Input: part model. Units: mm. Frame: model coordinates. A direction names the side the tool comes from. Round coordinates to 2 decimals unless told otherwise and drop trailing zeros. Loops run counter-clockwise (first coordinate to the right, second up) from the corner with the lowest first, then second, coordinate; pieces in that order, holes last.
1) First-contact query: pin 1 (0.9 mm diameter, centred on x = 0, y = 1, fed in from +Z); pin 2 (1 mm diameter, centred on x = 0.5, y = -1, fed in from +Z); pin 3 (0.9 mm diameter, centred on x = 0, y = -0.5, fed in from -Z); pin 4 (3 mm diameter, centred on y = -1, z = -1.5, fed in from +X). Flat tips, straight axial feed; report the tip coordinate or a pass-through.
2) Ray query, line 1 along Y through (x, z) = (0, -0.6); line 2 along Y through (x, z) = (-0.4, -1). Return the intervals inside material, ascending.
3) Section D-D, the plane z = -1. Return loops of the section in (x, y), and give its area (3 significant figures).
4) Access query for faces 5 (the face through (1, -0.7, 1.2)), 6 (the face through (-1, -0.7, 1.2)), 7 (the face through (-2.12, 1.17, 2.07)). Directions: +Z, -Z, +X, -X, +Y, -Y. A direction counts if a zero-diameter tool reaches every point of the face in a straight line with its end or side. Return the directions, or none.
5) Section C-C, the plane z = -2.5. Return loops of the section in (x, y).
6) Draft query along Y for faces 1 (the face through (2.07, 1.18, 2.03)), 2 (the face through (0, -1, 0)), 3 (the face through (0, 0, -1.2)), 4 (the face through (-0.323, 1.453, -1.446)). Return one class per face: pulls with the +Y half, pulls with the -Y half, needs draft (parallel to the pull), parting line crosses it, or undercut.
from build123d import *

# Parameters (mm, degrees)
SKETCH_R     = 1.5
SKETCH_R_2   = 1
PAD_DEPTH    = 1.2
SKETCH001_R  = 1.488237
PAD001_DEPTH = 0.5
SKETCH002_W  = 0.5
SKETCH002_H  = 2.7
PAD002_DEPTH = 0.25
SKETCH003_W  = 0.5
SKETCH003_H  = 3
PAD003_DEPTH = 0.25
PAD004_DEPTH = 0.25
PAD005_DEPTH = 0.25


with BuildPart() as part:
    # Sketch → Pad (new body, symmetric)
    with BuildSketch(Plane.XY):
        Circle(SKETCH_R)
        Circle(SKETCH_R_2, mode=Mode.SUBTRACT)
    extrude(amount=PAD_DEPTH, both=True)

    # Sketch001 (on Face3 of Pad) → Pad001 (join)
    with BuildSketch(Plane(origin=(0, 0, -1.2), x_dir=(1, 0, 0), z_dir=(0, 0, -1))):
        Circle(SKETCH001_R)
    extrude(amount=PAD001_DEPTH)

    # Sketch002 → Pad002 (join, symmetric)
    with BuildSketch(Plane.YZ):
        with Locations((0, -3.05)):
            Rectangle(SKETCH002_W, SKETCH002_H)
    extrude(amount=PAD002_DEPTH, both=True)

    # Sketch003 (on Face1 of CopyRuled_Surface) → Pad003 (join, symmetric)
    with BuildSketch(Plane(origin=(0, 0, 0), x_dir=(1, 0, 0), z_dir=(0, 0.707107, 0.707107))):
        with Locations((0, -2.9)):
            Rectangle(SKETCH003_W, SKETCH003_H)
    extrude(amount=PAD003_DEPTH, both=True)

    # Sketch004 (on CopyRuled_Surface) → Pad004 (join, symmetric)
    with BuildSketch(Plane(origin=(0, 0, 0), x_dir=(0.790569, -0.273861, 0.547723), z_dir=(0.612372, 0.353553, -0.707107))):
        Polygon((1.225119, -0.677557), (3.560833, -2.58466), (3.244606, -2.971958), (0.908891, -1.064855), align=None)
    extrude(amount=PAD004_DEPTH, both=True)

    # Sketch005 (on Face1 of CopyRuled_Surface002) → Pad005 (join, symmetric)
    with BuildSketch(Plane(origin=(0, 0, 0), x_dir=(0.790569, 0.273861, -0.547723), z_dir=(0.612372, -0.353553, 0.707107))):
        Polygon((-1.225119, 0.677557), (-3.560833, 2.58466), (-3.244606, 2.971958), (-0.908891, 1.064855), align=None)
    extrude(amount=PAD005_DEPTH, both=True)


solid = part.part
Final values:
1. pin 1: stops at z = 1.2
1. pin 2: stops at z = 1.79
1. pin 3: stops at z = -4.4
1. pin 4: stops at x = 1.5
2. line 1: y = -1.5 to -1, 1 to 1.5
2. line 2: y = -1.45 to -0.92, 0.92 to 1.45
3. outline: circle Ø3 at (0, 0); hole circle Ø2 at (0, 0)
3. area: 3.93 mm2
4. face 5: +Z, +X, -Y
4. face 6: +Z, -X, -Y
4. face 7: -Z, -X, +Y
5. outline: (-0.25, -0.25) - (0.25, -0.25) - (0.25, 0.25) - (-0.25, 0.25) - close
6. face 1: pulls with the +Y half
6. face 2: undercut
6. face 3: undercut
6. face 4: parting line crosses it
